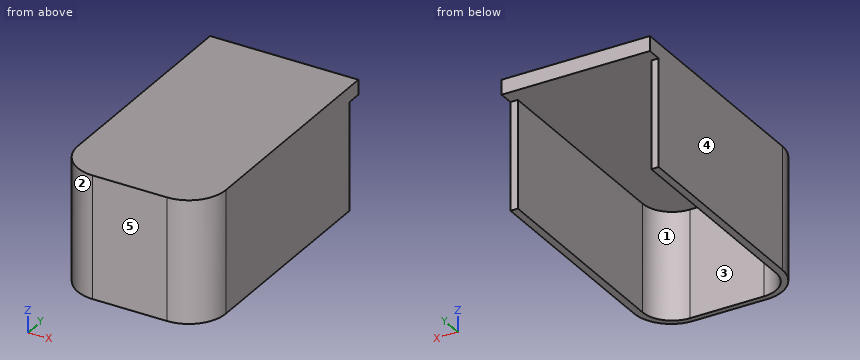
```python
from build123d import *

# Parameters (mm, degrees)
F1_DEPTH = 4
F2_DEPTH = 29


with BuildPart() as f1:
    # F0 (on Top) → F1 (new body)
    with BuildSketch(Plane.XY):
        with BuildLine():
            Line((-9.838484, -35.096727), (10.161516, -35.096727))
            ThreePointArc((10.161516, -35.096727), (17.232584, -32.167795), (20.161516, -25.096727))
            Line((20.161516, -25.096727), (20.161516, 30.903273))
            Line((20.161516, 30.903273), (18.161516, 30.903273))
            Line((18.161516, 30.903273), (18.161516, -25.596727))
            ThreePointArc((18.161516, -25.596727), (15.81837, -31.253582), (10.161516, -33.596727))
            Line((10.161516, -33.596727), (-9.838484, -33.596727))
            ThreePointArc((-9.838484, -33.596727), (-15.495338, -31.253582), (-17.838484, -25.596727))
            Line((-17.838484, -25.596727), (-17.838484, 30.903273))
            Line((-17.838484, 30.903273), (-19.838484, 30.903273))
            Line((-19.838484, 30.903273), (-19.838484, -25.096727))
            ThreePointArc((-19.838484, -25.096727), (-16.909552, -32.167795), (-9.838484, -35.096727))
        make_face()
        Polygon((18.161516, 30.903273), (20.161516, 30.903273), (20.161516, 34.903273), (-19.838484, 34.903273), (-19.838484, 30.903273), (-17.838484, 30.903273), (-16.838484, 30.903273), (-14.838484, 30.903273), (15.161516, 30.903273), (17.161516, 30.903273), align=None)
        with BuildLine():
            Line((18.161516, -25.596727), (18.161516, 30.903273))
            Line((18.161516, 30.903273), (17.161516, 30.903273))
            Line((17.161516, 30.903273), (17.161516, -25.596727))
            ThreePointArc((17.161516, -25.596727), (15.111263, -30.546475), (10.161516, -32.596727))
            Line((10.161516, -32.596727), (-9.838484, -32.596727))
            ThreePointArc((-9.838484, -32.596727), (-14.788231, -30.546475), (-16.838484, -25.596727))
            Line((-16.838484, -25.596727), (-16.838484, 30.903273))
            Line((-16.838484, 30.903273), (-17.838484, 30.903273))
            Line((-17.838484, 30.903273), (-17.838484, -25.596727))
            ThreePointArc((-17.838484, -25.596727), (-15.495338, -31.253582), (-9.838484, -33.596727))
            Line((-9.838484, -33.596727), (10.161516, -33.596727))
            ThreePointArc((10.161516, -33.596727), (15.81837, -31.253582), (18.161516, -25.596727))
        make_face()
        with BuildLine():
            Line((15.161516, -25.596727), (15.161516, 30.903273))
            Line((15.161516, 30.903273), (-14.838484, 30.903273))
            Line((-14.838484, 30.903273), (-14.838484, -25.596727))
            ThreePointArc((-14.838484, -25.596727), (-13.374018, -29.132261), (-9.838484, -30.596727))
            Line((-9.838484, -30.596727), (10.161516, -30.596727))
            ThreePointArc((10.161516, -30.596727), (13.69705, -29.132261), (15.161516, -25.596727))
        make_face()
        with BuildLine():
            Line((17.161516, -25.596727), (17.161516, 30.903273))
            Line((17.161516, 30.903273), (15.161516, 30.903273))
            Line((15.161516, 30.903273), (15.161516, -25.596727))
            ThreePointArc((15.161516, -25.596727), (13.69705, -29.132261), (10.161516, -30.596727))
            Line((10.161516, -30.596727), (-9.838484, -30.596727))
            ThreePointArc((-9.838484, -30.596727), (-13.374018, -29.132261), (-14.838484, -25.596727))
            Line((-14.838484, -25.596727), (-14.838484, 30.903273))
            Line((-14.838484, 30.903273), (-16.838484, 30.903273))
            Line((-16.838484, 30.903273), (-16.838484, -25.596727))
            ThreePointArc((-16.838484, -25.596727), (-14.788231, -30.546475), (-9.838484, -32.596727))
            Line((-9.838484, -32.596727), (10.161516, -32.596727))
            ThreePointArc((10.161516, -32.596727), (15.111263, -30.546475), (17.161516, -25.596727))
        make_face()
    extrude(amount=F1_DEPTH)

    # F0 (on Top) → F2 (join)
    with BuildSketch(Plane.XY):
        with BuildLine():
            Line((-9.838484, -35.096727), (10.161516, -35.096727))
            ThreePointArc((10.161516, -35.096727), (17.232584, -32.167795), (20.161516, -25.096727))
            Line((20.161516, -25.096727), (20.161516, 30.903273))
            Line((20.161516, 30.903273), (18.161516, 30.903273))
            Line((18.161516, 30.903273), (18.161516, -25.596727))
            ThreePointArc((18.161516, -25.596727), (15.81837, -31.253582), (10.161516, -33.596727))
            Line((10.161516, -33.596727), (-9.838484, -33.596727))
            ThreePointArc((-9.838484, -33.596727), (-15.495338, -31.253582), (-17.838484, -25.596727))
            Line((-17.838484, -25.596727), (-17.838484, 30.903273))
            Line((-17.838484, 30.903273), (-19.838484, 30.903273))
            Line((-19.838484, 30.903273), (-19.838484, -25.096727))
            ThreePointArc((-19.838484, -25.096727), (-16.909552, -32.167795), (-9.838484, -35.096727))
        make_face()
    extrude(amount=-F2_DEPTH)


solid = f1.part
```
Here's how the part is built. I have some questions about the finished solid (model axes, mm). Face numbers are marked on the shaded views. A direction names the side the tool comes from. Coordinates: 2 decimals unless noted, no trailing zeros. Order: outer loops, then holes, each group sorted by start corner. A loop starts at its lowest first (then second) coordinate and runs counter-clockwise, first axis right, second up. Notation, with made-up numbers: (-28, 52) -> (7, 52) arc R10 cw to (7, 59) -> close; hole circle Ø5 at (-30.75, -26.75). An arc over 180 degrees is marked (long way). Return JSON: item names as keys, results as strings.
1) If we section it at D-D on z = 2: List the corners of the cut face in (x, y) for me, plus the area to 3 significant figures.
Conclusion:
{"outline": "(-19.84, -25.1) arc R10 ccw to (-9.84, -35.1) -> (10.16, -35.1) arc R10 ccw to (20.16, -25.1) -> (20.16, 34.9) -> (-19.84, 34.9) -> close", "area": "2,760 mm²"}
2) If we section it at C-C on x = -0.5: List the corners of the cut face in (y, z) for me.
Conclusion:
{"outline": "(-35.1, -29) -> (-33.6, -29) -> (-33.6, 0) -> (34.9, 0) -> (34.9, 4) -> (-35.1, 4) -> close"}
3) I'm going to push flat-ended pins straight in: P1, Ø1, axis at x = -13, z = -11, coming from the +Y side; P2, Ø8, axis at x = 5.5, z = -24.5, coming from the +Y side; P3, Ø5, axis at x = -9.5, z = -17.5, coming from the +Y side. Where does each tip first touch, or does it pass through?
Conclusion:
{"P1": "stops at y = -32.71", "P2": "stops at y = -33.6", "P3": "stops at y = -33.3"}
4) If I drill on probe 1 along X at (y, z) = (2.5, -21.5); probe 2 along Z at (x, y) = (-16.5, 24.5); probe 3 along Y at (x, z) = (-9.5, -12), over which ranges is the centre line in solid material (lowest first)?
Conclusion:
{"probe 1": "x = -19.84 to -17.84, 18.16 to 20.16", "probe 2": "z = 0 to 4", "probe 3": "y = -35.1 to -33.6"}
5) If we section it at A-A on y = -20.5: List the corners of the cut face in (x, z) for me.
Conclusion:
{"outline": "(-19.84, -29) -> (-17.84, -29) -> (-17.84, 0) -> (18.16, 0) -> (18.16, -29) -> (20.16, -29) -> (20.16, 4) -> (-19.84, 4) -> close"}
6) On a 3-axis mill with a long thin cutter (end or side, diameter ignored), from which of +Z, -Z, +X, -X, +Y, -Y can I reach the whole of each face in a straight line? I mean the marked faces 1 and 2. Say none if no direction works.
Conclusion:
{"face 1": "-Z, +Y", "face 2": "+Z, -Z, -X, -Y"}
7) Thinking about a two-plate mould opening in X: for the marked faces 3, 4 and 5, which applies, +X half, -X half, draft (parallel to the pull), parting line (faces both ways), or undercut?
Conclusion:
{"face 3": "undercut", "face 4": "-X half", "face 5": "draft"}
8) If we section it at B-B on z = -25.5: List the corners of the cut face in (x, y) for me, plus the area to 3 significant figures.
Conclusion:
{"outline": "(-19.84, -25.1) arc R10 ccw to (-9.84, -35.1) -> (10.16, -35.1) arc R10 ccw to (20.16, -25.1) -> (20.16, 30.9) -> (18.16, 30.9) -> (18.16, -25.6) arc R8 cw to (10.16, -33.6) -> (-9.84, -33.6) arc R8 cw to (-17.84, -25.6) -> (-17.84, 30.9) -> (-19.84, 30.9) -> close", "area": "303 mm²"}
